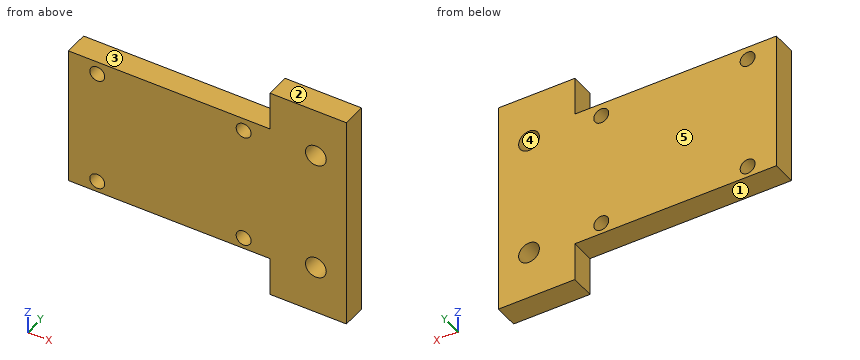
```python
from build123d import *

# Parameters (mm, degrees)
SKETCH1_R           = 2.159
SKETCH1_R_2         = 1.55
BOSS_EXTRUDE1_DEPTH = 5
SKETCH2_W           = 32.727568347
SKETCH2_H           = 13.013122107
SKETCH2_W_2         = 39.41277834
SKETCH2_H_2         = 24.474392352
CUT_EXTRUDE1_DEPTH  = 58.151492497


with BuildPart() as part:
    # Sketch1 → Boss-Extrude1 (new body)
    with BuildSketch(Plane(origin=(0, 0, 0), x_dir=(1, 0, 0), z_dir=(0, 1, 0))):
        Polygon((36.55, 27.14922), (36.55, -43.65078), (20.675, -43.65078), (20.675, -31.173955128), (-21.18269604, -31.173955128), (-21.18269604, -2.173955128), (20.675, -2.173955128), (20.675, 27.14922), align=None)
        with Locations(Location((30.2, -29.173955128, 0), (0, 0, 90))):
            Circle(SKETCH1_R, mode=Mode.SUBTRACT)
        with Locations(Location((-15.2, -28.50156, 0), (0, 0, 90))):
            Circle(SKETCH1_R_2, mode=Mode.SUBTRACT)
        with Locations(Location((15.19999, -28.50156, 0), (0, 0, 270))):
            Circle(SKETCH1_R_2, mode=Mode.SUBTRACT)
        with Locations(Location((-15.2, -4.50156, 0), (0, 0, 270))):
            Circle(SKETCH1_R_2, mode=Mode.SUBTRACT)
        with Locations(Location((15.2, -4.50156, 0), (0, 0, 90))):
            Circle(SKETCH1_R_2, mode=Mode.SUBTRACT)
        with Locations(Location((30.2, -4.173955128, 0), (0, 0, 270))):
            Circle(SKETCH1_R, mode=Mode.SUBTRACT)
    extrude(amount=BOSS_EXTRUDE1_DEPTH)

    # Sketch2 → Cut-Extrude1 (cut, through all)
    with BuildSketch(Plane(origin=(0, 5, 0), x_dir=(1, 0, 0), z_dir=(0, 1, 0))):
        with Locations((29.057065878, -45.680516182)):
            Rectangle(SKETCH2_W, SKETCH2_H)
        with Locations((32.399670874, 18.063241048)):
            Rectangle(SKETCH2_W_2, SKETCH2_H_2)
    extrude(amount=-CUT_EXTRUDE1_DEPTH, mode=Mode.SUBTRACT)


solid = part.part
```
For this review, take the finished solid that the model builds, in its own axes (mm). Face numbers are marked on the shaded views. A direction names the side the tool comes from. Coordinates: 2 decimals unless noted, no trailing zeros. Order: outer loops, then holes, each group sorted by start corner. A loop starts at its lowest first (then second) coordinate and runs counter-clockwise, first axis right, second up. Notation, with made-up numbers: (37.5, 35.5) - (79.5, 35.5) arc R29 ccw to (79.5, 58.5) - close; hole circle Ø8 at (87.5, 31). An arc over 180 degrees is marked (long way). Answer as a JSON object with one key per item and string values. Group by question number.
1. The part is to be moulded in two halves that separate along X. For the marked faces 4 and 5, say which applies: pulls with the +X half, pulls with the -X half, needs draft (parallel to the pull), parting line crosses it, or undercut.
2. Clearance check with flat-ended pins moving along their axes: P1, Ø1.5, axis at x = -6, y = 2.5, coming from the +Z side; P2, Ø1.5, axis at y = 1.5, z = -1.5, coming from the -X side (3 decimals); P3, Ø1, axis at x = 0, y = 1, coming from the -Z side. State where each tip first meets the part, or that it passes through.
3. We need section B-B on y = 4. State the section outline as (x, z) points (3 decimals), then the cut area to 3 significant figures.
4. For the marked faces 1, 2 and 3, list the 3-axis set-ups (+Z, -Z, +X, -X, +Y, -Y) from which the entire face can be reached by the end or side of a thin tool; tool diameter is ignored.
5. For probe 1 along Z at (x, y) = (14, 0.7); probe 2 along X at (y, z) = (1.6, 28.5); probe 3 along Z at (x, y) = (31.5, 0.8), list the stretches that pass through material, from the lowest coordinate up.
6. We need section A-A on x = 30.2. State the section outline as (y, z) points.
7. We need section D-D on z = 36. State the section outline as (x, y) points (3 decimals).
8. We need section C-C on x = -15.2. State the section outline as (y, z) points.
Final values:
{
 "1": {"face 4": "undercut", "face 5": "needs draft"},
 "2": {"P1": "z = 31.17", "P2": "x = 20.675", "P3": "z = 2.17"},
 "3": {"outline": "(-21.183, 2.174) - (20.675, 2.174) - (20.675, -5.826) - (36.55, -5.826) - (36.55, 39.174) - (20.675, 39.174) - (20.675, 31.174) - (-21.183, 31.174) - close; hole circle Ø3.1 at (-15.2, 4.502); hole circle Ø3.1 at (-15.2, 28.502); hole circle Ø3.1 at (15.2, 4.502); hole circle Ø3.1 at (15.2, 28.502); hole circle Ø4.318 at (30.2, 4.174); hole circle Ø4.318 at (30.2, 29.174)", "area": "1,870 mm²"},
 "4": {"face 1": "-Z, -X, +Y, -Y", "face 2": "+Z, +X, -X, +Y, -Y", "face 3": "+Z, -X, +Y, -Y"},
 "5": {"probe 1": "2.17 to 3.52, 5.48 to 27.52, 29.48 to 31.17", "probe 2": "-21.18 to -16.75, -13.65 to 13.65, 16.75 to 28.15, 32.25 to 36.55", "probe 3": "-5.83 to 2.45, 5.9 to 27.45, 30.9 to 39.17"},
 "6": {"outline": "(0, -5.83) - (5, -5.83) - (5, 2.01) - (0, 2.01) - close; (0, 6.33) - (5, 6.33) - (5, 27.01) - (0, 27.01) - close; (0, 31.33) - (5, 31.33) - (5, 39.17) - (0, 39.17) - close"},
 "7": {"outline": "(20.675, 0) - (36.55, 0) - (36.55, 5) - (20.675, 5) - close"},
 "8": {"outline": "(0, 2.17) - (5, 2.17) - (5, 2.95) - (0, 2.95) - close; (0, 6.05) - (5, 6.05) - (5, 26.95) - (0, 26.95) - close; (0, 30.05) - (5, 30.05) - (5, 31.17) - (0, 31.17) - close"}
}
